from build123d import *

# Parameters (mm, degrees)
BOSS_EXTRUDE1_DEPTH     = 20
SKETCH3_R               = 1.6375
CUT_EXTRUDE1_DEPTH      = 6
CUT_EXTRUDE1_DEPTH_BACK = 10
SKETCH7_R               = 2.05
CUT_EXTRUDE2_DEPTH      = 14
CUT_EXTRUDE2_DEPTH_BACK = 14


with BuildPart() as part:
    # Sketch1 → Boss-Extrude1 (new body)
    with BuildSketch(Plane(origin=(0, 0, 0), x_dir=(1, 0, 0), z_dir=(0, 1, 0))):
        Polygon((13, -5), (13, 9), (11, 9), (11, 2.5), (-11, 2.5), (-11, 9), (-13, 9), (-13, -5), align=None)
    extrude(amount=BOSS_EXTRUDE1_DEPTH)

    # Sketch3 → Cut-Extrude1 (cut, two sides)
    with BuildSketch(Plane.XY) as cut_extrude1_sk:
        with Locations((0, 10)):
            Circle(SKETCH3_R)
    extrude(amount=CUT_EXTRUDE1_DEPTH, mode=Mode.SUBTRACT)
    extrude(cut_extrude1_sk.sketch, amount=-CUT_EXTRUDE1_DEPTH_BACK, mode=Mode.SUBTRACT)

    # Sketch7 → Cut-Extrude2 (cut, two sides)
    with BuildSketch(Plane(origin=(0, 0, 0), x_dir=(0, 0, -1), z_dir=(1, 0, 0))) as cut_extrude2_sk:
        with Locations((5.75, 10)):
            Circle(SKETCH7_R)
    extrude(amount=CUT_EXTRUDE2_DEPTH, mode=Mode.SUBTRACT)
    extrude(cut_extrude2_sk.sketch, amount=-CUT_EXTRUDE2_DEPTH_BACK, mode=Mode.SUBTRACT)


solid = part.part
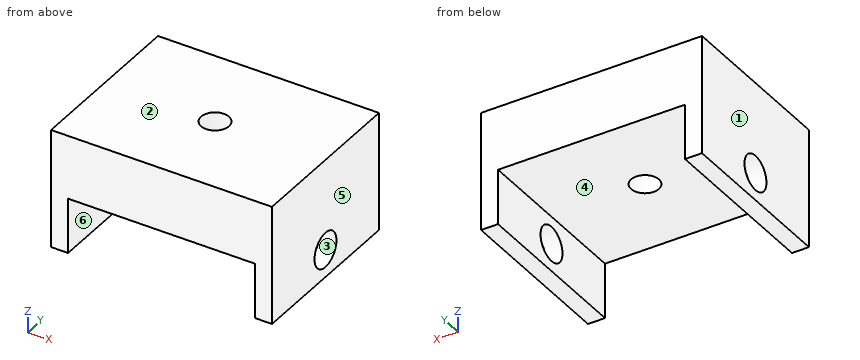
Verification items for the finished model (mm, model axes). Face numbers are marked on the shaded views. A direction names the side the tool comes from. Round coordinates to 2 decimals unless told otherwise and drop trailing zeros. Order: outer loops, then holes, each group sorted by start corner. A loop starts at its lowest first (then second) coordinate and runs counter-clockwise, first axis right, second up.
1. Section check D-D on y = 2.75. Record the cut outline in (x, z).
Final values:
outline: (-13, -9) - (-11, -9) - (-11, -2.5) - (11, -2.5) - (11, -9) - (13, -9) - (13, 5) - (-13, 5) - close
2. Release check for a two-part mould opening along Z. For the marked faces 1, 2, 3 and 4 record: +Z half, -Z half, draft (parallel to the pull), parting line (faces both ways), or undercut.
Final values:
face 1: draft
face 2: +Z half
face 3: undercut
face 4: -Z half
3. Go/stop test with flat-tipped pins: P1, Ø3, axis at x = -9, z = -5, coming from the +Y side; P2, Ø10, axis at x = -4.5, y = 12.5, coming from the -Z side; P3, Ø6, axis at x = -9, y = 17.5, coming from the -Z side. Record where each tip stops, or that it passes through.
Final values:
P1: passes through
P2: stops at z = -2.5
P3: stops at z = -9
4. Access from +Z, -Z, +X, -X, +Y, -Y to the whole of each face (thin tool, end or side, straight path). Record for the marked faces 5 and 6.
Final values:
face 5: +Z, -Z, +X, +Y, -Y
face 6: -Z, +Y, -Y
5. Thickness scan on L1, parallel to X at y = 5.25, z = -6.75; L2, parallel to Y at x = -12.2, z = -5.75; L3, parallel to Z at x = 12.15, y = 10. Record the ranges inside material, lowest first.
Final values:
L1: x = -13 to -11, 11 to 13
L2: y = 0 to 7.95, 12.05 to 20
L3: z = -9 to -7.8, -3.7 to 5
6. Section check B-B on z = -5.75. Record the cut outline in (x, y).
Final values:
outline: (-13, 0) - (-11, 0) - (-11, 7.95) - (-13, 7.95) - close; (-13, 12.05) - (-11, 12.05) - (-11, 20) - (-13, 20) - close; (11, 0) - (13, 0) - (13, 7.95) - (11, 7.95) - close; (11, 12.05) - (13, 12.05) - (13, 20) - (11, 20) - close
7. Section check A-A on y = 10. Record the cut outline in (x, z).
Final values:
outline: (-13, -9) - (-11, -9) - (-11, -7.8) - (-13, -7.8) - close; (-13, -3.7) - (-11, -3.7) - (-11, -2.5) - (-1.64, -2.5) - (-1.64, 5) - (-13, 5) - close; (1.64, -2.5) - (11, -2.5) - (11, -3.7) - (13, -3.7) - (13, 5) - (1.64, 5) - close; (11, -9) - (13, -9) - (13, -7.8) - (11, -7.8) - close
8. Section check C-C on x = 0. Record the cut outline in (y, z), then the cut area to 3 significant figures.
Final values:
outline: (0, -2.5) - (8.36, -2.5) - (8.36, 5) - (0, 5) - close; (11.64, -2.5) - (20, -2.5) - (20, 5) - (11.64, 5) - close
area: 125 mm2
